Build history of the part. All positions in model axes, mm. A direction names the side the tool comes from. Give positions to 0.01 mm unless a question says otherwise; leave off trailing zeros. Write each loop counter-clockwise with the first axis right and the second up, starting at its lowest first coordinate (ties: lowest second). Pieces come first, ordered by that corner, then holes.
from build123d import *

# Parameters (mm, degrees)
ESQUISSE1_R             = 3.25
BOSS_EXTRU_1_DEPTH      = 10
CONG_1_R                = 5
CONG_2_R                = 3
ESQUISSE2_R             = 6
ENL_V_MAT_EXTRU_1_DEPTH = 1.5
ESQUISSE3_R             = 2.65
ENL_V_MAT_EXTRU_2_DEPTH = 13


with BuildPart() as part:
    # Esquisse1 → Boss.-Extru.1 (new body, symmetric)
    with BuildSketch(Plane.XY):
        Polygon((0, 0), (-15.265735364, 0), (-16.548069585, -7), (-28.548069585, -7), (-28.548069585, 5), (0, 5), align=None)
        with Locations((-22, -1)):
            Circle(ESQUISSE1_R, mode=Mode.SUBTRACT)
    boss_extru_1 = extrude(amount=BOSS_EXTRU_1_DEPTH, both=True)

    # Symétrie1: Boss.-Extru.1 across plane
    add(boss_extru_1.mirror(Plane(origin=(0, 5, 10), x_dir=(0, 0, 1), z_dir=(-1, 0, 0))))

    # Congé1
    cong_1_edges = [part.edges().sort_by_distance(p)[0] for p in [
        (-15.265735364, 0, 0),
        (-28.548069585, -7, 0),
        (-28.548069585, 5, 0),
        (15.265735364, 0, 0),
        (28.548069585, -7, 0),
        (28.548069585, 5, 0),
    ]]
    fillet(cong_1_edges, radius=CONG_1_R)

    # Congé2
    cong_2_edges = [part.edges().sort_by_distance(p)[0] for p in [
        (-16.548069585, -7, 0),
        (16.548069585, -7, 0),
    ]]
    fillet(cong_2_edges, radius=CONG_2_R)

    # Esquisse2 → Enlèv. mat.-Extru.1 (cut)
    with BuildSketch(Plane.XZ):
        Circle(ESQUISSE2_R)
    extrude(amount=-ENL_V_MAT_EXTRU_1_DEPTH, mode=Mode.SUBTRACT)

    # Esquisse3 → Enlèv. mat.-Extru.2 (cut, through all)
    with BuildSketch(Plane(origin=(0, 5, 0), x_dir=(1, 0, 0), z_dir=(0, 1, 0))):
        Circle(ESQUISSE3_R)
    extrude(amount=-ENL_V_MAT_EXTRU_2_DEPTH, mode=Mode.SUBTRACT)


solid = part.part
(1) Probe line 1 (Z direction, x = 0, y = 0.8); line 2 (X direction, y = 0.5, z = 8.5); line 3 (Y direction, x = 22, z = -3.25). List the from-to ranges inside material, lowest first.
(2) Saw through at C-C, the plane y = -1. List the corners of the cut face in (x, z), plus the area to 3 significant figures.
(3) 3-axis set-ups, long thin cutter, end or side, ignore diameter. For faces 4 (the face through (3, 1.5, -1)), 5 (the face through (-5, 0, -4)), 6 (the face through (25.247, -0.857, -0.14)): which of +Z, -Z, +X, -X, +Y, -Y reach the whole face in a straight line?
(4) Mould opens along X. For faces 1 (the face through (27.045, 3.574, 0.14)), 2 (the face through (-25.247, -0.857, -0.14)), 3 (the face through (-0.4, 0.4, 10)) say: +X half, -X half, draft (parallel to the pull), parting line (faces both ways), or undercut.
(5) Saw through at B-B, the plane z = 0. List the corners of the cut face in (x, y).
(6) Saw through at D-D, the plane z = 7.5. List the corners of the cut face in (x, y), plus the area to 3 significant figures.
(7) Drop flat-ended pins along their axis: pin 1 (6 mm diameter, centred on y = -5.5, z = -0.5, fed in from -X); pin 2 (3 mm diameter, centred on x = 0, z = 0, fed in from -Y); pin 3 (6 mm diameter, centred on x = -2.5, z = 1, fed in from -Y); pin 4 (3 mm diameter, centred on y = 2, z = 7.5, fed in from +X). Give the stop position or say it passes through.
(8) Saw through at A-A, the plane x = -22. List the corners of the cut face in (y, z).
Computed values:
1. line 1: z = -10 to -6, 6 to 10
1. line 2: x = -28.52 to -24.88, -19.12 to 19.12, 24.88 to 28.52
1. line 3: y = -7 to -4.25, 2.25 to 5
2. outline: (-28.55, -10) - (-25.25, -10) - (-25.25, 10) - (-28.55, 10) - close; (-18.75, -10) - (-14.1, -10) - (-14.1, 10) - (-18.75, 10) - close; (14.1, -10) - (18.75, -10) - (18.75, 10) - (14.1, 10) - close; (25.25, -10) - (28.55, -10) - (28.55, 10) - (25.25, 10) - close
2. area: 318 mm2
3. face 4: -Y
3. face 5: +Z, -Z, -Y
3. face 6: +Z, -Z
4. face 1: +X half
4. face 2: undercut
4. face 3: draft
5. outline: (-28.55, -2) arc R5 ccw to (-23.55, -7) - (-19.05, -7) arc R3 ccw to (-16.1, -4.54) - (-16.02, -4.1) arc R5 cw to (-11.1, 0) - (-6, 0) - (-6, 1.5) - (-2.65, 1.5) - (-2.65, 5) - (-23.55, 5) arc R5 ccw to (-28.55, 0) - close; (2.65, 1.5) - (6, 1.5) - (6, 0) - (11.1, 0) arc R5 cw to (16.02, -4.1) - (16.1, -4.54) arc R3 ccw to (19.05, -7) - (23.55, -7) arc R5 ccw to (28.55, -2) - (28.55, 0) arc R5 ccw to (23.55, 5) - (2.65, 5) - close; hole circle Ø6.5 at (-22, -1); hole circle Ø6.5 at (22, -1)
6. outline: (-28.55, -2) arc R5 ccw to (-23.55, -7) - (-19.05, -7) arc R3 ccw to (-16.1, -4.54) - (-16.02, -4.1) arc R5 cw to (-11.1, 0) - (11.1, 0) arc R5 cw to (16.02, -4.1) - (16.1, -4.54) arc R3 ccw to (19.05, -7) - (23.55, -7) arc R5 ccw to (28.55, -2) - (28.55, 0) arc R5 ccw to (23.55, 5) - (-23.55, 5) arc R5 ccw to (-28.55, 0) - close; hole circle Ø6.5 at (-22, -1); hole circle Ø6.5 at (22, -1)
6. area: 379 mm2
7. pin 1: stops at x = -28.52
7. pin 2: passes through
7. pin 3: stops at y = 1.5
7. pin 4: stops at x = 28.52
8. outline: (-7, -10) - (-4.25, -10) - (-4.25, 10) - (-7, 10) - close; (2.25, -10) - (5, -10) - (5, 10) - (2.25, 10) - close
